Can you work these out from the model? Positions are in its coordinate system, mm. Face numbers are marked on the shaded views. A direction names the side the tool comes from. Coordinates: 2 decimals unless noted, no trailing zeros. Loops run counter-clockwise (first coordinate to the right, second up) from the corner with the lowest first, then second, coordinate; pieces in that order, holes last. Notation, with made-up numbers: (71, -8.5) -> (108, -8.5) arc R25 cw to (108, 3.5) -> close; hole circle Ø8 at (51, -9.5). An arc over 180 degrees is marked (long way). Use one line per item in the form item = value. Start each with the question number.
(1) I'm going to push flat-ended pins straight in: pin 1 (2 mm diameter, centred on x = 34, y = 11, fed in from +Z); pin 2 (6 mm diameter, centred on y = 31, z = 21, fed in from -X); pin 3 (6 mm diameter, centred on x = 8.5, z = 12.5, fed in from +Y). Where does each tip first touch, or does it pass through?
(2) Imagine slicing it at C-C (y = 23.5). List the corners of the cut face in (x, z) for me.
(3) Imagine slicing it at D-D (x = 26). List the corners of the cut face in (y, z) for me, plus the area to 3 significant figures.
(4) Thinking about a two-plate mould opening in Y: for the marked faces 4, 5 and 6, which applies, released by +Y, released by -Y, zero draft, split by the parting line, or undercut?
(5) On a 3-axis mill with a long thin cutter (end or side, diameter ignored), from which of +Z, -Z, +X, -X, +Y, -Y can I reach the whole of each face in a straight line? I mean the marked faces 1, 2 and 3. Say none if no direction works.
(6) I need wall thicknesses on line 1 (X direction, y = 33, z = 21.5); line 2 (Z direction, x = 20, y = 8). Which ranges of each line are inside material? Lowest first, please. Write a range as [from, to].
(7) Imagine slicing it at A-A (x = 35). List the corners of the cut face in (y, z) for me, plus the area to 3 significant figures.
(8) Imagine slicing it at B-B (z = 3). List the corners of the cut face in (x, y) for me.
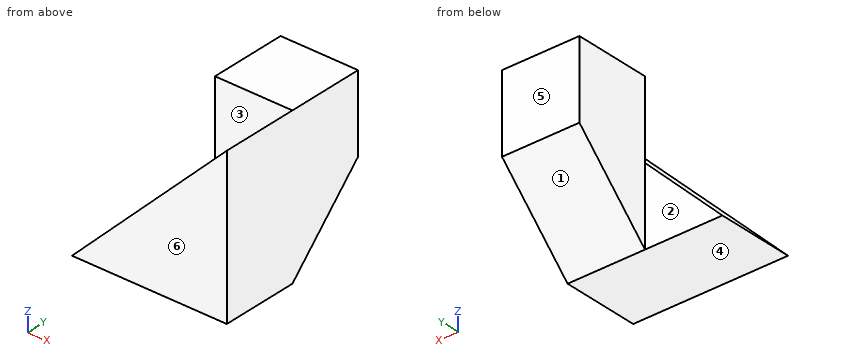
```python
from build123d import *

# Parameters (mm, degrees)
SKETCH1_W           = 40
SKETCH1_H           = 20
BOSS_EXTRUDE1_DEPTH = 40
CUT_EXTRUDE1_DEPTH  = 40
SKETCH3_W           = 40
SKETCH3_H           = 20
BOSS_EXTRUDE2_DEPTH = 20
CUT_EXTRUDE2_DEPTH  = 20


with BuildPart() as part:
    # Sketch1 → Boss-Extrude1 (new body)
    with BuildSketch(Plane.XY):
        with Locations((20, 10)):
            Rectangle(SKETCH1_W, SKETCH1_H)
    extrude(amount=BOSS_EXTRUDE1_DEPTH)

    # Sketch2 → Cut-Extrude1 (cut)
    with BuildSketch(Plane(origin=(0, 20, 0), x_dir=(1, 0, 0), z_dir=(0, 1, 0))):
        Polygon((0, 0), (40, -40), (0, -40), align=None)
    extrude(amount=-CUT_EXTRUDE1_DEPTH, mode=Mode.SUBTRACT)

    # Sketch3 → Boss-Extrude2 (add)
    with BuildSketch(Plane(origin=(40, 0, 0), x_dir=(0, 0, -1), z_dir=(1, 0, 0))):
        with Locations((-20, 30)):
            Rectangle(SKETCH3_W, SKETCH3_H)
    extrude(amount=-BOSS_EXTRUDE2_DEPTH)

    # Sketch4 → Cut-Extrude2 (cut)
    with BuildSketch(Plane.ZY.offset(-20)):
        Polygon((0, 20), (20, 40), (0, 40), align=None)
    extrude(amount=-CUT_EXTRUDE2_DEPTH, mode=Mode.SUBTRACT)


solid = part.part
```
Worked out:
q1.pin_1 = 35
q1.pin_2 = 20
q1.pin_3 = 20
q2.outline = (20, 3.5) -> (40, 3.5) -> (40, 40) -> (20, 40) -> close
q3.outline = (0, 0) -> (20, 0) -> (40, 20) -> (40, 40) -> (20, 40) -> (20, 26) -> (0, 26) -> close
q3.area = 1,120 mm2
q4.face_4 = zero draft
q4.face_5 = released by +Y
q4.face_6 = released by -Y
q5.face_1 = -Z, +X, -X, +Y
q5.face_2 = +Z, -Z, -X, +Y
q5.face_3 = +Z, -X, -Y
q6.line_1 = [20, 40]
q6.line_2 = [0, 20]
q7.outline = (0, 0) -> (20, 0) -> (40, 20) -> (40, 40) -> (20, 40) -> (20, 35) -> (0, 35) -> close
q7.area = 1,300 mm2
q8.outline = (3, 0) -> (40, 0) -> (40, 23) -> (20, 23) -> (20, 20) -> (3, 20) -> close
